Source: CAD feature listing. Evaluate the final solid. Frame: model axes, mm. Face numbers are marked on the shaded views. A direction names the side the tool comes from. Give positions to 0.01 mm unless a question says otherwise; leave off trailing zeros. Order: outer loops, then holes, each group sorted by start corner. A loop starts at its lowest first (then second) coordinate and runs counter-clockwise, first axis right, second up. Notation, with made-up numbers: (14, 4) - (66, 4) arc R22 cw to (66, 26) - close; hole circle Ø9 at (56.25, -22). An arc over 180 degrees is marked (long way). Use CSV: the item, a comma, the result in double quotes.
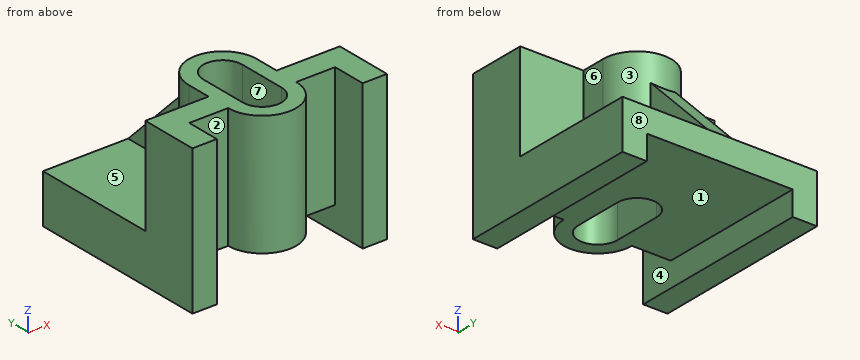
```python
from build123d import *

# Parameters (mm, degrees)
BOSS_EXTRUDE1_DEPTH = 20
SKETCH2_W           = 30
SKETCH2_H           = 7
CUT_EXTRUDE1_DEPTH  = 31
BOSS_EXTRUDE3_DEPTH = 30
CUT_EXTRUDE2_DEPTH  = 31
SKETCH5_W           = 30
SKETCH5_H           = 5
CUT_EXTRUDE3_DEPTH  = 39
RIB2_REACH          = 22
SKETCH6_WALL_W      = 61.798989874
SKETCH6_WALL_H      = 5


with BuildPart() as part:
    # Sketch1 → Boss-Extrude1 (new body, symmetric)
    with BuildSketch(Plane(origin=(0, 0, 0), x_dir=(0, 0, -1), z_dir=(1, 0, 0))):
        Polygon((0, 38), (0, 0), (-30, 0), (-30, 12), (-10, 12), (-10, 38), align=None)
    extrude(amount=BOSS_EXTRUDE1_DEPTH, both=True)

    # Sketch2 → Cut-Extrude1 (cut, through all)
    with BuildSketch(Plane.XY.offset(30)):
        with Locations((0, 3.5)):
            Rectangle(SKETCH2_W, SKETCH2_H)
    extrude(amount=-CUT_EXTRUDE1_DEPTH, mode=Mode.SUBTRACT)

    # Sketch3 → Boss-Extrude3 (add)
    with BuildSketch(Plane.XY.offset(30)):
        with BuildLine():
            Line((7, 17), (7, 7))
            ThreePointArc((7, 7), (0, 0), (-7, 7))
            Line((-7, 7), (-7, 17))
            ThreePointArc((-7, 17), (0, 24), (7, 17))
        make_face()
    extrude(amount=-BOSS_EXTRUDE3_DEPTH)

    # Sketch4 → Cut-Extrude2 (cut, through all)
    with BuildSketch(Plane.XY.offset(30)):
        with BuildLine():
            Line((4, 17), (4, 7))
            ThreePointArc((4, 7), (0, 3), (-4, 7))
            Line((-4, 7), (-4, 17))
            ThreePointArc((-4, 17), (0, 21), (4, 17))
        make_face()
    extrude(amount=-CUT_EXTRUDE2_DEPTH, mode=Mode.SUBTRACT)

    # Sketch5 → Cut-Extrude3 (cut, through all)
    with BuildSketch(Plane(origin=(0, 38, 0), x_dir=(1, 0, 0), z_dir=(0, 1, 0))):
        with Locations((0, -2.5)):
            Rectangle(SKETCH5_W, SKETCH5_H)
    extrude(amount=-CUT_EXTRUDE3_DEPTH, mode=Mode.SUBTRACT)

    # Sketch6 wall → Rib2 (add, up to next)
    with BuildSketch(Plane(origin=(0, 31, 17), x_dir=(0, -0.707106781, 0.707106781), z_dir=(0, -0.707106781, -0.707106781)), mode=Mode.PRIVATE) as rib2_sk1:
        Rectangle(SKETCH6_WALL_W, SKETCH6_WALL_H)
    rib2_tool1 = extrude(rib2_sk1.sketch, amount=RIB2_REACH, mode=Mode.PRIVATE) - part.part
    add(rib2_tool1.solids().sort_by_distance((0, 31, 17))[0])


solid = part.part
```
Item 1: Section B-B on z = 26.5. Return the cut outline in (x, y).
Filled in:
outline,"(-20, 0) - (-15, 0) - (-15, 7) - (-7, 7) arc R7 ccw to (7, 7) - (15, 7) - (15, 0) - (20, 0) - (20, 12) - (7, 12) - (7, 17) arc R7 ccw to (-7, 17) - (-7, 12) - (-20, 12) - close; hole (-4, 7) arc R4 ccw to (4, 7) - (4, 17) arc R4 ccw to (-4, 17) - close"
Item 2: Section D-D on z = 19. Return the cut outline in (x, y), then the cut area to 3 significant figures.
Filled in:
outline,"(-20, 0) - (-15, 0) - (-15, 7) - (-7, 7) arc R7 ccw to (7, 7) - (15, 7) - (15, 0) - (20, 0) - (20, 12) - (7, 12) - (7, 17) arc R7 ccw to (2.5, 23.54) - (2.5, 29) - (-2.5, 29) - (-2.5, 23.54) arc R7 ccw to (-7, 17) - (-7, 12) - (-20, 12) - close; hole (-4, 7) arc R4 ccw to (4, 7) - (4, 17) arc R4 ccw to (-4, 17) - close"
area,"389 mm2"
Item 3: Set-up query: the marked faces 1, 2, 3, 4 and 5. Return all of +Z, -Z, +X, -X, +Y, -Y with unobstructed straight access to the full face (end or side cutting, diameter ignored); none if empty.
Filled in:
face 1,"-Z, +Y, -Y"
face 2,"+Z, -Z, -Y"
face 3,"+Z, +Y"
face 4,"-Z, -Y"
face 5,"+Z, -X, +Y"
Item 4: Section A-A on x = 0. Return the cut outline in (y, z).
Filled in:
outline,"(0, 5) - (3, 5) - (3, 30) - (0, 30) - close; (21, 5) - (38, 5) - (38, 10) - (24, 24) - (24, 30) - (21, 30) - close"
Item 5: First-contact query: pin 1 (3 mm diameter, centred on y = 22, z = 17.5, fed in from +X); pin 2 (10 mm diameter, centred on x = -12.5, y = 29, fed in from +Z); pin 3 (6 mm diameter, centred on x = -2.5, y = 25, fed in from -Z). Flat tips, straight axial feed; report the tip coordinate or a pass-through.
Filled in:
pin 1,"stops at x = 6.06"
pin 2,"stops at z = 10"
pin 3,"stops at z = 5"
Item 6: Material intervals for line 1 (X direction, y = 17, z = 18.25); line 2 (X direction, y = 6, z = 12.25); line 3 (X direction, y = 23.5, z = 2.75), sorted ascending. Write a range as from..to.
Filled in:
line 1,"x = -7..-4, 4..7"
line 2,"x = -20..-15, -6.93..-3.87, 3.87..6.93, 15..20"
line 3,"x = -20..-15, 15..20"
Item 7: Section C-C on y = 8. Return the cut outline in (x, z).
Filled in:
outline,"(-20, 0) - (-15, 0) - (-15, 5) - (-4, 5) - (-4, 30) - (-20, 30) - close; (4, 5) - (15, 5) - (15, 0) - (20, 0) - (20, 30) - (4, 30) - close"
Item 8: Mould query, pull axis Y, two halves, no side actions, for the marked faces 6, 7 and 8. Classes: released by +Y, released by -Y, zero draft, split by the parting line, or undercut.
Filled in:
face 6,"zero draft"
face 7,"undercut"
face 8,"released by +Y"
